from build123d import *

# Parameters (mm, degrees)
SKETCH1_R           = 3
SKETCH1_R_2         = 1.5
BOSS_EXTRUDE1_DEPTH = 3
CUT_EXTRUDE1_DEPTH  = 3
CIRPATTERN1_COUNT   = 5


with BuildPart() as part:
    # Sketch1 → Boss-Extrude1 (new body)
    with BuildSketch(Plane(origin=(0, 0, 0), x_dir=(1, 0, 0), z_dir=(0, 1, 0))):
        with Locations(Location((0, 0, 0), (0, 0, 270))):
            Circle(SKETCH1_R)
        with Locations(Location((0, 0, 0), (0, 0, 270))):
            Circle(SKETCH1_R_2, mode=Mode.SUBTRACT)
    extrude(amount=BOSS_EXTRUDE1_DEPTH)

    # Sketch2 → Cut-Extrude1 (cut)
    with BuildSketch(Plane(origin=(0, 0, 0), x_dir=(0, 0, -1), z_dir=(1, 0, 0))):
        with BuildLine():
            ThreePointArc((0, 2), (-0.5, 1.5), (0, 1))
            Line((0, 1), (0, 2))
        make_face()
        with BuildLine():
            Line((0, 2), (0, 1))
            ThreePointArc((0, 1), (0.353553391, 1.146446609), (0.5, 1.5))
            ThreePointArc((0.5, 1.5), (0.353553391, 1.853553391), (0, 2))
        make_face()
    cut_extrude1 = extrude(amount=-CUT_EXTRUDE1_DEPTH, mode=Mode.SUBTRACT)

    # CirPattern1: Cut-Extrude1 ×5 about axis
    cirpattern1_axis = Axis((0, 0, 0), (0, 1, 0))
    for i in range(1, CIRPATTERN1_COUNT):
        add(cut_extrude1.rotate(cirpattern1_axis, i * 360 / CIRPATTERN1_COUNT), mode=Mode.SUBTRACT)


solid = part.part
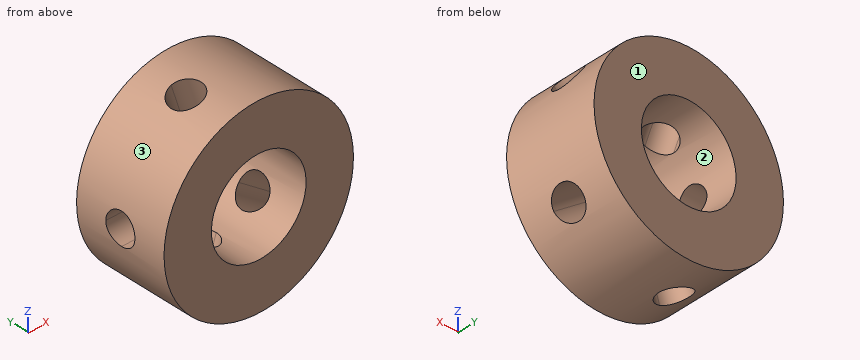
Work out the finished part from the listing and answer in its coordinate system (mm). Face numbers are marked on the shaded views. Give positions to 0.01 mm unless a question says otherwise; leave off trailing zeros. Loops run counter-clockwise (first coordinate to the right, second up) from the corner with the lowest first, then second, coordinate; pieces in that order, holes last. Notation, with made-up numbers: (-37.5, -24) -> (16.5, -24) arc R13 ccw to (16.5, -16) -> close; hole circle Ø5 at (89.5, 56). An arc over 180 degrees is marked (long way). Use a Markdown table: item, result. Add a question column.
1) This flat-tipped pin is pushed along its axis until it touches: P1, Ø2.5, axis at x = 0, z = 0, coming from the +Y side. Where does it stop, or does it pass through?
2) The part is cut by section B-B, the plane y = 2.5. Determine the outline of the cut face in (x, z).
3) Consider line 1 along X through (y, z) = (0.75, 0); line 2 along X through (y, z) = (1.7, 0); line 3 along Z through (x, y) = (-1, 2.5). Determine where each line is inside the solid, lowest interval first.
4) The part is cut by section A-A, the plane x = -2. Determine the outline of the cut face in (y, z), plus the area to 3 significant figures.
5) For a pull along Z with two mould halves and no side action, classify the marked faces 1, 2 and 3 as +Z half, -Z half, draft (parallel to the pull), parting line (faces both ways), or undercut.
6) The part is cut by section C-C, the plane z = -0.25. Determine the outline of the cut face in (x, y), plus the area to 3 significant figures.
7) The part is cut by section D-D, the plane y = 1.1. Determine the outline of the cut face in (x, z), plus the area to 3 significant figures.
Reported:
| question | item | result |
|---|---|---|
| 1 | P1 | passes through |
| 2 | outline | circle Ø6 at (0, 0); hole circle Ø3 at (0, 0) |
| 3 | line 1 | x = -3 to -1.5, 1.5 to 3 |
| 3 | line 2 | x = 1.5 to 3 |
| 3 | line 3 | z = -2.83 to -1.12, 1.12 to 2.83 |
| 4 | outline | (0, -2.24) -> (3, -2.24) -> (3, 2.24) -> (0, 2.24) -> close; hole circle Ø1 at (1.5, 0) |
| 4 | area | 12.6 mm^2 |
| 5 | face 1 | draft |
| 5 | face 2 | undercut |
| 5 | face 3 | parting line |
| 6 | outline | (-2.99, 0) -> (-1.48, 0) -> (-1.48, 1.07) -> (-2.99, 1.07) -> close; (-2.99, 1.93) -> (-1.48, 1.93) -> (-1.48, 3) -> (-2.99, 3) -> close; (1.48, 0) -> (2.99, 0) -> (2.99, 3) -> (1.48, 3) -> close |
| 6 | area | 7.76 mm^2 |
| 7 | outline | (-2.98, -0.3) arc R3 ccw to (-1.21, -2.75) -> (-0.74, -1.31) arc R1.5 cw to (-1.47, -0.3) -> close; (-2.98, 0.3) -> (-1.47, 0.3) arc R1.5 cw to (-0.74, 1.31) -> (-1.21, 2.75) arc R3 ccw to start; (-0.64, -2.93) arc R3 ccw to (2.24, -2) -> (1.01, -1.11) arc R1.5 cw to (-0.17, -1.49) -> close; (-0.64, 2.93) -> (-0.17, 1.49) arc R1.5 cw to (1.01, 1.11) -> (2.24, 2) arc R3 ccw to start; (1.37, -0.62) -> (2.59, -1.51) arc R3 ccw to (2.59, 1.51) -> (1.37, 0.62) arc R1.5 cw to start |
| 7 | area | 16.7 mm^2 |
